Verification items for this drawing (mm, ordinates from the low corner). A direction names the side the tool comes from. Give positions to 0.01 mm unless a question says otherwise; leave off trailing zeros. Write each loop counter-clockwise with the first axis right and the second up, starting at its lowest first coordinate (ties: lowest second). Pieces come first, ordered by that corner, then holes. Notation, with made-up numbers: (61.25, 65.25) -> (86.25, 65.25) arc R15 cw to (86.25, 71.25) -> close; hole circle Ø8 at (46.5, 54.25). An arc over 180 degrees is marked (long way). One line per item, written item: value.
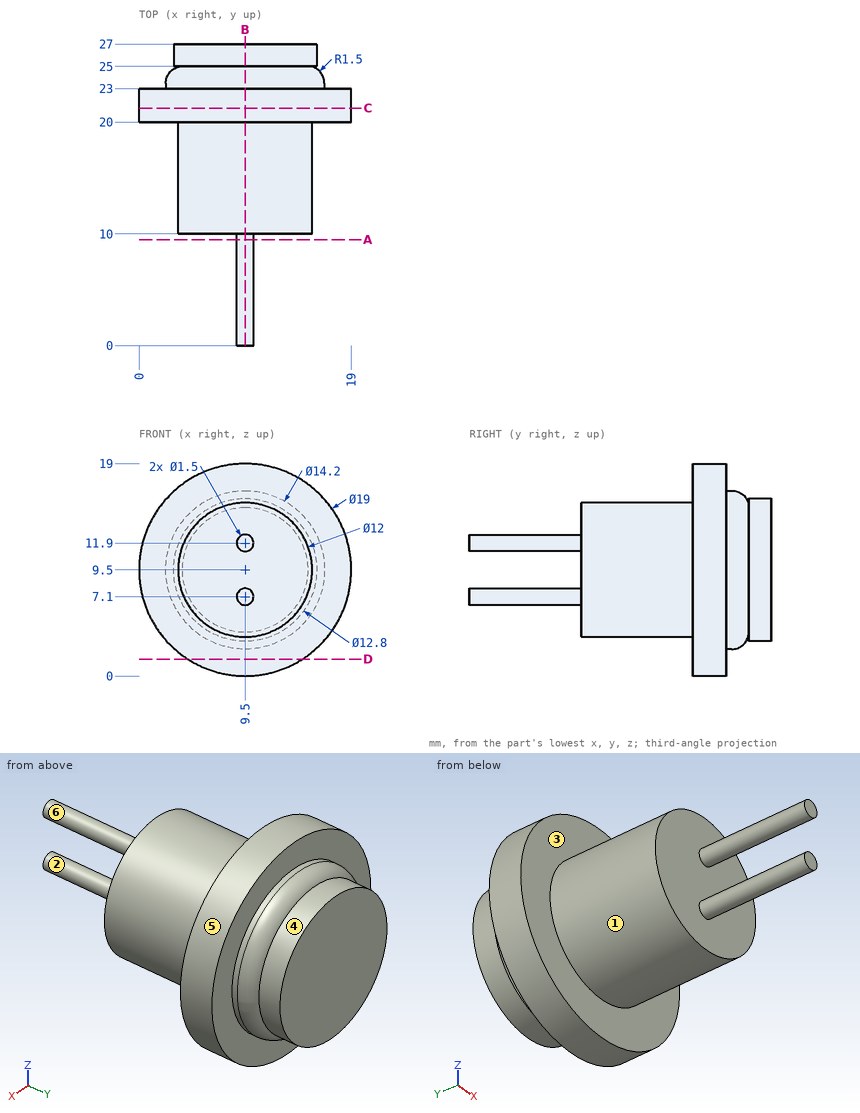
1) Tool access check on the marked faces 4, 5 and 6. Record the directions out of +Z, -Z, +X, -X, +Y, -Y that give a thin tool (end or side, any length) a straight path to the whole face; none if there is none.
Verdict:
face 4: +Y
face 5: +Y, -Y
face 6: -Y
2) Sectioned sample at A-A on y = 9.5. Record the cut outline in (x, z), plus the area to 3 significant figures.
Verdict:
outline: circle Ø1.5 at (9.5, 7.1); circle Ø1.5 at (9.5, 11.9)
area: 3.53 mm^2
3) Mould release check, pull along Z, two halves, no side actions. Record for the marked faces 1, 2 and 3: released by +Z, released by -Z, zero draft, split by the parting line, or undercut.
Verdict:
face 1: split by the parting line
face 2: undercut
face 3: zero draft
4) Depth check by flat-ended pin: pin 1 Ø3 at (x, y) = (14, 17.5) entering from -Z; pin 2 Ø3 at (y, z) = (7.5, 13.5) entering from +X; pin 3 Ø1.5 at (x, z) = (8.5, 9.5) entering from -Y. Enter the tip coordinate at first touch or a pass-through.
Verdict:
pin 1: z = 4.3
pin 2: x = 10.24
pin 3: y = 10
5) Sectioned sample at C-C on y = 21.25. Record the cut outline in (x, z), plus the area to 3 significant figures.
Verdict:
outline: circle Ø19 at (9.5, 9.5)
area: 284 mm^2
6) Scan lines: probe 1 along Y at (x, z) = (16.75, 5.75); probe 2 along Z at (x, y) = (10, 1.5); probe 3 along Y at (x, z) = (10.75, 8.75). Record each from-to range of solid material in increasing order.
Verdict:
probe 1: 20 to 23
probe 2: 6.54 to 7.66, 11.34 to 12.46
probe 3: 10 to 27
7) Sectioned sample at B-B on x = 9.5. Record the cut outline in (y, z), plus the area to 3 significant figures.
Verdict:
outline: (0, 6.35) -> (10, 6.35) -> (10, 3.5) -> (20, 3.5) -> (20, 0) -> (23, 0) -> (23, 2.4) -> (23.5, 2.4) arc R1.5 ccw to (25, 3.9) -> (25, 3.1) -> (27, 3.1) -> (27, 15.9) -> (25, 15.9) -> (25, 15.1) arc R1.5 ccw to (23.5, 16.6) -> (23, 16.6) -> (23, 19) -> (20, 19) -> (20, 15.5) -> (10, 15.5) -> (10, 12.65) -> (0, 12.65) -> (0, 11.15) -> (10, 11.15) -> (10, 7.85) -> (0, 7.85) -> close
area: 260 mm^2
8) Sectioned sample at D-D on z = 1.5. Record the cut outline in (x, y), plus the area to 3 significant figures.
Verdict:
outline: (4.38, 20) -> (14.62, 20) -> (14.62, 23) -> (4.38, 23) -> close
area: 30.7 mm^2
